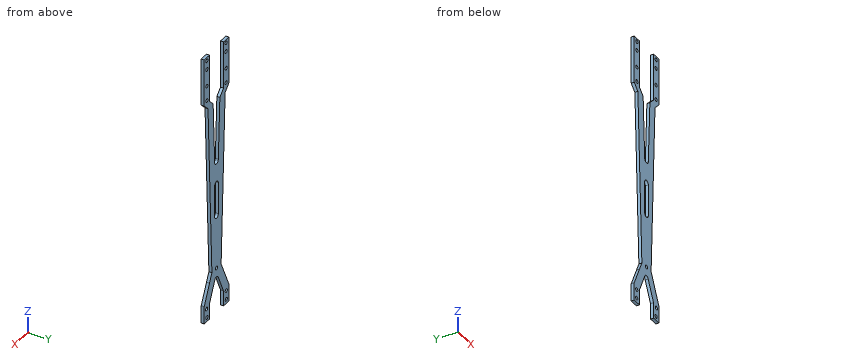
from build123d import *

# Parameters (mm, degrees)
SKETCH1_W           = 33.8
SKETCH1_H           = 228.6
BOSS_EXTRUDE1_DEPTH = 2.5
CUT_EXTRUDE1_DEPTH  = 2.5
SKETCH2_6_OUTSIDE_W = 82.02
SKETCH2_6_OUTSIDE_H = 276.82
CUT_EXTRUDE2_DEPTH  = 2.5
SKETCH5_R           = 1.5
CUT_EXTRUDE3_DEPTH  = 2.5


with BuildPart() as part:
    # Sketch1 → Boss-Extrude1 (new body)
    with BuildSketch(Plane(origin=(0, 0, 0), x_dir=(1, 0, 0), z_dir=(0, 1, 0))):
        with Locations((16.9, 114.3)):
            Rectangle(SKETCH1_W, SKETCH1_H)
    extrude(amount=BOSS_EXTRUDE1_DEPTH)

    # Sketch2 → Cut-Extrude1 (cut)
    with BuildSketch(Plane(origin=(0, 2.5, 0), x_dir=(1, 0, 0), z_dir=(0, 1, 0))):
        with BuildLine():
            Line((14.4, 144.5), (14.4, 117.5))
            add(Edge.make_bspline(
                [(14.4, 117.5), (14.399430285, 117.132237239), (14.536831695, 116.524171276), (14.991581605, 115.839645543), (15.586717627, 115.318158312), (16.441592425, 114.966926324), (17.439533495, 114.99714129), (18.330206262, 115.381489106), (19.143348717, 116.172968782), (19.401576387, 116.99766646), (19.4, 117.5)],
                knots=[0, 0, 0, 0, 0.141327045, 0.23205331, 0.31123598, 0.442337735, 0.576355834, 0.682960692, 0.808345553, 1, 1, 1, 1], degree=3))
            Line((19.4, 117.5), (19.4, 144.5))
            add(Edge.make_bspline(
                [(14.4, 144.5), (14.395253504, 145.223790204), (14.991433849, 146.512706872), (16.62609513, 147.107640812), (17.903590827, 146.872098871), (19.022537404, 146.103569848), (19.403497366, 145.098391499), (19.4, 144.5)],
                knots=[0, 0, 0, 0, 0.27696704, 0.498348678, 0.612918932, 0.769853345, 1, 1, 1, 1], degree=3))
        make_face()
    extrude(amount=-CUT_EXTRUDE1_DEPTH, mode=Mode.SUBTRACT)

    # Sketch2_6 outside → Cut-Extrude2 (cut)
    with BuildSketch(Plane(origin=(0, 2.5, 0), x_dir=(1, 0, 0), z_dir=(0, 1, 0))):
        with Locations((16.9, 114.3)):
            Rectangle(SKETCH2_6_OUTSIDE_W, SKETCH2_6_OUTSIDE_H)
        with BuildLine():
            Line((0, 228.6), (7.25, 228.6))
            Line((7.25, 228.6), (7.25, 215.6))
            Line((7.25, 215.6), (14.582490059, 199.162371251))
            add(Edge.make_bspline(
                [(14.582490059, 199.162371251), (14.711561898, 198.842062842), (15.023836131, 198.378588046), (15.614972661, 197.928802428), (16.251883656, 197.646972571), (17.023429753, 197.553241488), (17.859761798, 197.743006401), (18.671860535, 198.240651313), (19.070795177, 198.798035014), (19.217509941, 199.162371251)],
                knots=[0, 0, 0, 0, 0.175078363, 0.276949723, 0.373162948, 0.525807757, 0.662070379, 0.801161333, 1, 1, 1, 1], degree=3))
            Line((19.217509941, 199.162371251), (26.55, 215.173869546))
            Line((26.55, 215.173869546), (26.55, 228.6))
            Line((26.55, 228.6), (33.8, 228.6))
            Line((33.8, 228.6), (33.8, 213.6))
            Line((33.8, 213.6), (26.55, 197.6))
            Line((26.55, 197.6), (23.25, 190.35))
            Line((23.25, 190.35), (28.588836909, 45.211163091))
            Line((28.588836909, 45.211163091), (33.8, 40))
            Line((33.8, 40), (33.8, 0))
            Line((33.8, 0), (26.55, 0))
            Line((26.55, 0), (26.55, 40))
            Line((26.55, 40), (21.55, 45))
            Line((21.55, 45), (19.4, 97.5))
            add(Edge.make_bspline(
                [(14.4, 97.5), (14.39963006, 97.808675141), (14.484997073, 98.261085854), (14.753428782, 98.807348646), (15.054139544, 99.215057311), (15.586652418, 99.681982141), (16.380265598, 100.007326678), (17.208278255, 100.01514461), (17.857989388, 99.833449339), (18.395045275, 99.537224279), (18.85030775, 99.106523366), (19.272621439, 98.433524922), (19.400681372, 97.867995006), (19.4, 97.5)],
                knots=[0, 0, 0, 0, 0.118087348, 0.173138637, 0.232058356, 0.311090992, 0.441944339, 0.550747407, 0.622172143, 0.698428615, 0.783497697, 0.859367045, 1, 1, 1, 1], degree=3))
            Line((14.4, 97.5), (12.25, 45))
            Line((12.25, 45), (7.25, 40))
            Line((7.25, 40), (7.25, 0))
            Line((7.25, 0), (0, 0))
            Line((0, 0), (0, 40))
            Line((0, 40), (5, 45))
            Line((5, 45), (10.53515625, 190.35))
            Line((10.53515625, 190.35), (7.23515625, 197.632758621))
            Line((7.23515625, 197.632758621), (0, 213.6))
            Line((0, 213.6), (0, 228.6))
        make_face(mode=Mode.SUBTRACT)
    extrude(amount=-CUT_EXTRUDE2_DEPTH, mode=Mode.SUBTRACT)

    # Sketch5 → Cut-Extrude3 (cut)
    with BuildSketch(Plane(origin=(0, 2.5, 0), x_dir=(1, 0, 0), z_dir=(0, 1, 0))):
        with Locations(Location((3.398371539, 225.1, 0), (0, 0, 270))):
            Circle(SKETCH5_R)
        with Locations(Location((30.132823035, 225.1, 0), (0, 0, 270))):
            Circle(SKETCH5_R)
        with Locations(Location((30.468201459, 217.6, 0), (0, 0, 270))):
            Circle(SKETCH5_R)
        with Locations(Location((3.398371539, 217.6, 0), (0, 0, 270))):
            Circle(SKETCH5_R)
        with Locations(Location((3.625, 37.333121102, 0), (0, 0, 270))):
            Circle(SKETCH5_R)
        with Locations(Location((30.175, 37.333121102, 0), (0, 0, 270))):
            Circle(SKETCH5_R)
        with Locations(Location((30.175, 24.833121102, 0), (0, 0, 270))):
            Circle(SKETCH5_R)
        with Locations(Location((3.625, 24.833121102, 0), (0, 0, 270))):
            Circle(SKETCH5_R)
        with Locations(Location((3.625, 10.333121102, 0), (0, 0, 270))):
            Circle(SKETCH5_R)
        with Locations(Location((3.625, 2.833121102, 0), (0, 0, 270))):
            Circle(SKETCH5_R)
        with Locations(Location((30.175, 2.833121102, 0), (0, 0, 270))):
            Circle(SKETCH5_R)
        with Locations(Location((30.175, 10.333121102, 0), (0, 0, 270))):
            Circle(SKETCH5_R)
        with Locations(Location((16.926550078, 190.1, 0), (0, 0, 270))):
            Circle(SKETCH5_R)
    extrude(amount=-CUT_EXTRUDE3_DEPTH, mode=Mode.SUBTRACT)


solid = part.part
Geometry: final body of the model. Coordinates: model frame, mm. Coordinates: 2 decimals unless noted, no trailing zeros. Order: outer loops, then holes, each group sorted by start corner. A loop starts at its lowest first (then second) coordinate and runs counter-clockwise, first axis right, second up.
(1) Material intervals for probe 1 along X at (y, z) = (1.9, -225.1); probe 2 along X at (y, z) = (1.4, -31.5); probe 3 along Z at (x, y) = (18, 1.65), sorted ascending.
(2) First-contact query: pin 1 (4 mm diameter, centred on x = 3.62, z = -24.83, fed in from +Y). Flat tip, straight axial feed; report the tip coordinate or a pass-through.
(3) Section query A-A (z = -90). Return the cut outline in (x, y), plus the area to 3 significant figures.
(4) Section query B-B (y = 0.65). State how many separate pieces and enclosed holes the cut face has, plus the area to 3 significant figures.
Solution:
1. probe 1: x = 0 to 1.9, 4.9 to 7.25, 26.55 to 28.63, 31.63 to 33.8
1. probe 2: x = 0 to 7.25, 26.55 to 33.8
1. probe 3: z = -197.86 to -191.15, -189.05 to -146.74, -115.25 to -99.74
2. pin 1: stops at y = 2.5
3. outline: (6.71, 0) - (14.09, 0) - (14.09, 2.5) - (6.71, 2.5) - close; (19.71, 0) - (26.94, 0) - (26.94, 2.5) - (19.71, 2.5) - close
3. area: 36.5 mm2
4. separate pieces: 1
4. enclosed holes: 14
4. area: 3,250 mm2
